Verification items for the finished model (mm, model axes). A direction names the side the tool comes from. Give positions to 0.01 mm unless a question says otherwise; leave off trailing zeros. Order: outer loops, then holes, each group sorted by start corner. A loop starts at its lowest first (then second) coordinate and runs counter-clockwise, first axis right, second up. Notation, with made-up numbers: M -25.5,83.5 L 29.5,83.5 A19 cw 29.5,93.5 Z; hole C 85.25,-10 d5. An arc over 180 degrees is marked long. Answer as a JSON object with one key per item and string values.
```python
from build123d import *

# Parameters (mm, degrees)
EXTRUDE_1_DEPTH     = 12
EXTRUDE_2_DEPTH     = 4
CUT_EXTRUDE_1_REACH = 107.216
SKETCH_3_R          = 1.6
CUT_EXTRUDE_2_REACH = 107.216
SKETCH_4_R          = 1.6
FILLET_2_R          = 2
SKETCH_5_W          = 11.2
SKETCH_5_H          = 20
CUT_EXTRUDE_3_DEPTH = 20
FILLET_4_R          = 2


with BuildPart() as part:
    # Sketch 1 → Extrude 1 (new body)
    with BuildSketch(Plane.XY):
        Polygon((42.5, 0), (0, 0), (0, 42.5), (3, 42.5), (3, 3), (42.5, 3), align=None)
    extrude(amount=EXTRUDE_1_DEPTH)

    # Sketch 1_6 → Extrude 2 (add)
    with BuildSketch(Plane.XY):
        with BuildLine():
            Line((95.5, 42.5), (3, 42.5))
            Line((3, 42.5), (3, 3))
            Line((3, 3), (42.5, 3))
            Line((42.5, 3), (53.5, 3))
            ThreePointArc((53.5, 3), (57.035533906, 4.464466094), (58.5, 8))
            Line((58.5, 8), (58.5, 20.5))
            ThreePointArc((58.5, 20.5), (61.428932188, 27.571067812), (68.5, 30.5))
            Line((68.5, 30.5), (95.5, 30.5))
            Line((95.5, 30.5), (95.5, 42.5))
        make_face()
        with BuildLine():
            ThreePointArc((28, 29.5), (28.585786438, 30.914213562), (30, 31.5))
            Line((30, 31.5), (42, 31.5))
            ThreePointArc((42, 31.5), (43.414213562, 30.914213562), (44, 29.5))
            Line((44, 29.5), (44, 13.5))
            ThreePointArc((44, 13.5), (43.414213562, 12.085786438), (42, 11.5))
            Line((42, 11.5), (30, 11.5))
            ThreePointArc((30, 11.5), (28.585786438, 12.085786438), (28, 13.5))
            Line((28, 13.5), (28, 29.5))
        make_face(mode=Mode.SUBTRACT)
    extrude(amount=EXTRUDE_2_DEPTH)

    # Sketch 3 → Cut-Extrude 1 (cut, up to next)
    with BuildSketch(Plane.ZY, mode=Mode.PRIVATE) as cut_extrude_1_sk1:
        with Locations((8, 10.5)):
            Circle(SKETCH_3_R)
    cut_extrude_1_tool1 = extrude(cut_extrude_1_sk1.sketch, amount=-CUT_EXTRUDE_1_REACH, mode=Mode.PRIVATE) & part.part
    # Sketch 3 → Cut-Extrude 1 (cut, up to next)
    with BuildSketch(Plane.ZY, mode=Mode.PRIVATE) as cut_extrude_1_sk2:
        with Locations((8, 34.5)):
            Circle(SKETCH_3_R)
    cut_extrude_1_tool2 = extrude(cut_extrude_1_sk2.sketch, amount=-CUT_EXTRUDE_1_REACH, mode=Mode.PRIVATE) & part.part
    add(cut_extrude_1_tool1.solids().sort_by_distance((0, 10.5, 8))[0], mode=Mode.SUBTRACT)
    add(cut_extrude_1_tool2.solids().sort_by_distance((0, 34.5, 8))[0], mode=Mode.SUBTRACT)

    # Sketch 4 → Cut-Extrude 2 (cut, up to next)
    with BuildSketch(Plane.XZ, mode=Mode.PRIVATE) as cut_extrude_2_sk1:
        with Locations((10.5, 8)):
            Circle(SKETCH_4_R)
    cut_extrude_2_tool1 = extrude(cut_extrude_2_sk1.sketch, amount=-CUT_EXTRUDE_2_REACH, mode=Mode.PRIVATE) & part.part
    # Sketch 4 → Cut-Extrude 2 (cut, up to next)
    with BuildSketch(Plane.XZ, mode=Mode.PRIVATE) as cut_extrude_2_sk2:
        with Locations((34.5, 8)):
            Circle(SKETCH_4_R)
    cut_extrude_2_tool2 = extrude(cut_extrude_2_sk2.sketch, amount=-CUT_EXTRUDE_2_REACH, mode=Mode.PRIVATE) & part.part
    add(cut_extrude_2_tool1.solids().sort_by_distance((10.5, 0, 8))[0], mode=Mode.SUBTRACT)
    add(cut_extrude_2_tool2.solids().sort_by_distance((34.5, 0, 8))[0], mode=Mode.SUBTRACT)

    # Fillet 2
    fillet_2_edges = [part.edges().sort_by_distance(p)[0] for p in [
        (42.5, 1.5, 12),
        (1.5, 42.5, 12),
        (42.5, 1.5, 0),
    ]]
    fillet(fillet_2_edges, radius=FILLET_2_R)

    # Mirror 1: part across plane


with BuildPart() as part_1:
    add(part.part)
    add(part.part.mirror(Plane(origin=(95.5, 0, 4), x_dir=(0, 0, 1), z_dir=(-1, 0, 0))))

    # Sketch 5 → Cut-Extrude 3 (cut)
    with BuildSketch(Plane.XY.offset(4)):
        with Locations((47.6, 21.5)):
            Rectangle(SKETCH_5_W, SKETCH_5_H)
        with Locations((143.4, 21.5)):
            Rectangle(SKETCH_5_W, SKETCH_5_H)
    extrude(amount=-CUT_EXTRUDE_3_DEPTH, mode=Mode.SUBTRACT)

    # Fillet 4
    fillet_4_edges = [part_1.edges().sort_by_distance(p)[0] for p in [
        (53.2, 11.5, 2),
        (53.2, 31.5, 2),
        (137.8, 11.5, 2),
        (137.8, 31.5, 2),
    ]]
    fillet(fillet_4_edges, radius=FILLET_4_R)


solid = part_1.part
```
Q1. Section check B-B on y = 18. Record the cut outline in (x, z), then the cut area to 3 significant figures.
Resolved:
{"outline": "M 0,0 L 28,0 L 28,4 L 3,4 L 3,12 L 0,12 Z; M 53.2,0 L 58.5,0 L 58.5,4 L 53.2,4 Z; M 132.5,0 L 137.8,0 L 137.8,4 L 132.5,4 Z; M 163,0 L 191,0 L 191,12 L 188,12 L 188,4 L 163,4 Z", "area": "314 mm²"}
Q2. Section check D-D on x = 118.5. Record the cut outline in (y, z).
Resolved:
{"outline": "M 30.5,0 L 42.5,0 L 42.5,4 L 30.5,4 Z"}
Q3. Gauge pin test, flat ends, axial feed: pin 1 Ø4 at (x, z) = (10.5, 8) entering from +Y; pin 2 Ø2 at (x, z) = (142.5, 2.5) entering from -Y; pin 3 Ø12 at (x, y) = (59.5, 13.5) entering from +Z. Record the tip position at first contact, or that the pin passes through.
Resolved:
{"pin 1": "stops at y = 3", "pin 2": "stops at y = 3", "pin 3": "stops at z = 4"}
Q4. Release check for a two-part mould opening along Z. For faces 5 (the face through (47, 3, 2)), 6 (the face through (97, 31, 0)), 7 (the face through (8.9, 1.48, 8.07)) record: +Z half, -Z half, draft (parallel to the pull), parting line (faces both ways), or undercut.
Resolved:
{"face 5": "draft", "face 6": "-Z half", "face 7": "undercut"}
Q5. Section check C-C on x = 34.5. Record the cut outline in (y, z).
Resolved:
{"outline": "M 0,0 L 11.5,0 L 11.5,4 L 3,4 L 3,6.4 L 0,6.4 Z; M 0,9.6 L 3,9.6 L 3,12 L 0,12 Z; M 31.5,0 L 42.5,0 L 42.5,4 L 31.5,4 Z"}
Q6. Section check A-A on y = 34.5. Record the cut outline in (x, z), then the cut area to 3 significant figures.
Resolved:
{"outline": "M 0,0 L 191,0 L 191,6.4 L 188,6.4 L 188,4 L 3,4 L 3,6.4 L 0,6.4 Z; M 0,9.6 L 3,9.6 L 3,12 L 0,12 Z; M 188,9.6 L 191,9.6 L 191,12 L 188,12 Z", "area": "793 mm²"}
Q7. Tool access check on faces 1 (the face through (188, 23, 8)), 2 (the face through (132.5, 14, 2)), 3 (the face through (28, 21, 2)), 4 (the face through (94, 42.5, 2)). Record the directions out of +Z, -Z, +X, -X, +Y, -Y that give a thin tool (end or side, any length) a straight path to the whole face; none if there is none.
Resolved:
{"face 1": "+Z, +Y", "face 2": "+Z, -Z, -Y", "face 3": "+Z, -Z", "face 4": "+Z, -Z, +X, -X, +Y"}
Q8. Material ranges on L1, parallel to X at y = 14, z = 3.5; L2, parallel to X at y = 33.5, z = 9.5; L3, parallel to Y at x = 2.15, z = 8, recorded low to high.
Resolved:
{"L1": "x = 0 to 28, 53.2 to 58.5, 132.5 to 137.8, 163 to 191", "L2": "x = 0 to 3, 188 to 191", "L3": "y = 0 to 8.9, 12.1 to 32.9, 36.1 to 42.5"}
